Check sheet for the modelled part. Datum: model origin and axes. Units: mm. Face numbers are marked on the shaded views. A direction names the side the tool comes from. Round coordinates to 2 decimals unless told otherwise and drop trailing zeros. Write each loop counter-clockwise with the first axis right and the second up, starting at its lowest first coordinate (ties: lowest second). Pieces come first, ordered by that corner, then holes. Notation, with made-up numbers: M -17,22 L 32,22 A15 ccw 32,37 Z; hole C 63.5,36.25 d5. An arc over 180 degrees is marked long. Answer in a Markdown table with one row per item.
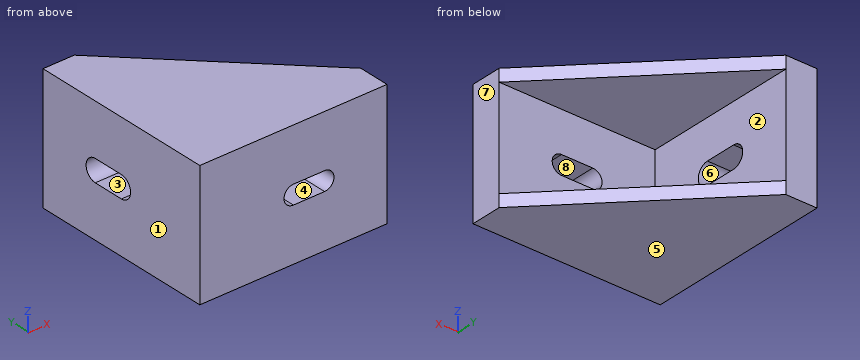
```python
from build123d import *

# Parameters (mm, degrees)
EXTRUDE_1_DEPTH     = 20
SKETCH_3_W          = 16
SKETCH_3_H          = 25
CUT_EXTRUDE_1_DEPTH = 25
CUT_EXTRUDE_2_REACH = 45.875
CUT_EXTRUDE_3_REACH = 45.875


with BuildPart() as part:
    # 草圖1 → 填料-伸長1 (new body)
    with BuildSketch(Plane.XY):
        Polygon((0, 0), (0, -30), (30, -30), (30, -25), (5, 0), align=None)
    extrude(amount=-EXTRUDE_1_DEPTH)

    # 草圖3 → 除料-伸長1 (cut)
    with BuildSketch(Plane(origin=(30, 0, 0), x_dir=(0, 0, -1), z_dir=(1, 0, 0))):
        with Locations((10, -12.5)):
            Rectangle(SKETCH_3_W, SKETCH_3_H)
    extrude(amount=-CUT_EXTRUDE_1_DEPTH, mode=Mode.SUBTRACT)

    # 草圖4 → 除料-伸長2 (cut, up to next)
    with BuildSketch(Plane(origin=(5, 0, 0), x_dir=(0, 0, -1), z_dir=(1, 0, 0)), mode=Mode.PRIVATE) as cut_extrude_2_sk1:
        with BuildLine():
            Line((11.75, -10), (11.75, -15))
            ThreePointArc((11.75, -15), (10, -16.75), (8.25, -15))
            Line((8.25, -15), (8.25, -10))
            ThreePointArc((8.25, -10), (10, -8.25), (11.75, -10))
        make_face()
    cut_extrude_2_tool1 = extrude(cut_extrude_2_sk1.sketch, amount=-CUT_EXTRUDE_2_REACH, mode=Mode.PRIVATE) & part.part
    add(cut_extrude_2_tool1.solids().sort_by_distance((5, -12.5, -10))[0], mode=Mode.SUBTRACT)

    # 草圖5 → 除料-伸長3 (cut, up to next)
    with BuildSketch(Plane(origin=(0, -25, 0), x_dir=(1, 0, 0), z_dir=(0, 1, 0)), mode=Mode.PRIVATE) as cut_extrude_3_sk1:
        with BuildLine():
            Line((15, 11.5), (20, 11.5))
            ThreePointArc((20, 11.5), (21.5, 10), (20, 8.5))
            Line((20, 8.5), (15, 8.5))
            ThreePointArc((15, 8.5), (13.5, 10), (15, 11.5))
        make_face()
    cut_extrude_3_tool1 = extrude(cut_extrude_3_sk1.sketch, amount=-CUT_EXTRUDE_3_REACH, mode=Mode.PRIVATE) & part.part
    add(cut_extrude_3_tool1.solids().sort_by_distance((17.5, -25, -10))[0], mode=Mode.SUBTRACT)


solid = part.part
```
1. Go/stop test with a flat-tipped pin: pin 1 (6 mm diameter, centred on x = 20, z = -7.5, fed in from +Y). Record where the tip stops, or that it passes through.
Found:
| item | result |
|---|---|
| pin 1 | stops at y = -25 |
2. Access from +Z, -Z, +X, -X, +Y, -Y to the whole of each face (thin tool, end or side, straight path). Record for the marked faces 1, 2, 3 and 4.
Found:
| item | result |
|---|---|
| face 1 | +Z, -Z, -X, +Y, -Y |
| face 2 | +X, +Y |
| face 3 | +X, -X |
| face 4 | +Y, -Y |
3. Scan lines: L1, parallel to Z at x = 18.5, y = -24.5; L2, parallel to Z at x = 19.25, y = -25.5; L3, parallel to Y at x = 23.25, z = -12.5. Record each from-to range of solid material in increasing order.
Found:
| item | result |
|---|---|
| L1 | z = -20 to -18, -2 to 0 |
| L2 | z = -20 to -11.5, -8.5 to 0 |
| L3 | y = -30 to -25 |
4. Section check A-A, the plane z = -10. Record the cut outline in (x, y), and give its area (4 significant figures).
Found:
| item | result |
|---|---|
| outline | M 0,-30 L 13.5,-30 L 13.5,-25 L 5,-25 L 5,-16.75 L 0,-16.75 Z; M 0,-8.25 L 5,-8.25 L 5,0 L 0,0 Z; M 21.5,-30 L 30,-30 L 30,-25 L 21.5,-25 Z |
| area | 192.5 mm2 |
5. Draft check along Z on the marked faces 5, 6, 7 and 8. Enter one of: +Z half, -Z half, draft (parallel to the pull), parting line (faces both ways), or undercut.
Found:
| item | result |
|---|---|
| face 5 | -Z half |
| face 6 | undercut |
| face 7 | draft |
| face 8 | undercut |
6. Section check C-C, the plane x = 25.75. Record the cut outline in (y, z).
Found:
| item | result |
|---|---|
| outline | M -30,-20 L -20.75,-20 L -20.75,-18 L -25,-18 L -25,-2 L -20.75,-2 L -20.75,0 L -30,0 Z |
7. Section check B-B, the plane x = 17.5. Record the cut outline in (y, z), and give its area (3 significant figures).
Found:
| item | result |
|---|---|
| outline | M -30,-20 L -12.5,-20 L -12.5,-18 L -25,-18 L -25,-11.5 L -30,-11.5 Z; M -30,-8.5 L -25,-8.5 L -25,-2 L -12.5,-2 L -12.5,0 L -30,0 Z |
| area | 135 mm2 |
8. Section check D-D, the plane y = -17.5. Record the cut outline in (x, z).
Found:
| item | result |
|---|---|
| outline | M 0,-20 L 22.5,-20 L 22.5,-18 L 5,-18 L 5,-2 L 22.5,-2 L 22.5,0 L 0,0 Z |
